Geometry check sheet. Reference: the model listing, model coordinates, mm. Face numbers are marked on the shaded views. Give positions to 0.01 mm unless a question says otherwise; leave off trailing zeros. Loops run counter-clockwise (first coordinate to the right, second up) from the corner with the lowest first, then second, coordinate; pieces in that order, holes last.
1. Release check for a two-part mould opening along Z. For the marked faces 1, 2 and 3 record: +Z half, -Z half, draft (parallel to the pull), parting line (faces both ways), or undercut.
2. Material ranges on L1, parallel to Z at x = -1.25, y = -1.7; L2, parallel to X at y = -4.65, z = -1.75; L3, parallel to Z at x = 0, y = -3.35, recorded low to high.
3. Cross-section at B-B, the plane x = 0. Record the cut outline in (y, z), plus the area to 3 significant figures.
4. Go/stop test with flat-tipped pins: pin 1 Ø2 at (y, z) = (-1, -8.5) entering from -X; pin 2 Ø3 at (y, z) = (-4.5, 7) entering from +X; pin 3 Ø3 at (y, z) = (-2.5, -2) entering from -X. Record where each tip stops, or that it passes through.
5. Cross-section at A-A, the plane z = 0. Record the cut outline in (x, y), plus the area to 3 significant figures.
6. Cross-section at C-C, the plane y = -1.35. Record the cut outline in (x, z), plus the area to 3 significant figures.
7. Cross-section at D-D, the plane y = -5.15. Record the cut outline in (x, z).
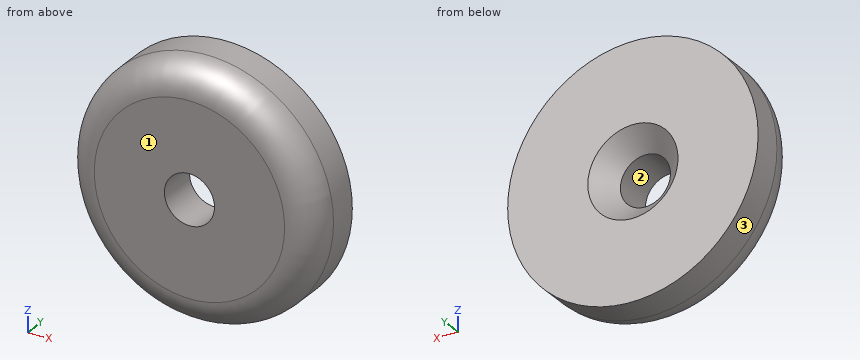
from build123d import *

# Parameters (mm, degrees)
F0_R     = 12.5
F0_R_2   = 2.5
F1_DEPTH = 6
F2_R     = 3
F3_SIZE  = 2


with BuildPart() as f1:
    # F0 (on Front) → F1 (new body)
    with BuildSketch(Plane.XZ):
        Circle(F0_R)
        Circle(F0_R_2, mode=Mode.SUBTRACT)
    extrude(amount=F1_DEPTH)

    # F2
    f2_edges = [f1.edges().sort_by_distance(p)[0] for p in [
        (-12.5, -6, 0),
    ]]
    fillet(f2_edges, radius=F2_R)

    # F3
    f3_edges = [f1.edges().sort_by_distance(p)[0] for p in [
        (-2.5, 0, 0),
    ]]
    chamfer(f3_edges, length=F3_SIZE)


solid = f1.part
Result:
1. face 1: draft
1. face 2: undercut
1. face 3: parting line
2. L1: z = -12.44 to -2.51, 2.51 to 12.44
2. L2: x = -11.88 to -1.79, 1.79 to 11.88
2. L3: z = -12.48 to -2.5, 2.5 to 12.48
3. outline: (-6, -9.5) arc R3 ccw to (-3, -12.5) - (0, -12.5) - (0, -4.5) - (-2, -2.5) - (-6, -2.5) - close; (-6, 2.5) - (-2, 2.5) - (0, 4.5) - (0, 12.5) - (-3, 12.5) arc R3 ccw to (-6, 9.5) - close
3. area: 112 mm2
4. pin 1: stops at x = -10
4. pin 2: stops at x = 11.02
4. pin 3: stops at x = -12.49
5. outline: (-12.5, -3) arc R3 ccw to (-9.5, -6) - (-2.5, -6) - (-2.5, -2) - (-4.5, 0) - (-12.5, 0) - close; (2.5, -6) - (9.5, -6) arc R3 ccw to (12.5, -3) - (12.5, 0) - (4.5, 0) - (2.5, -2) - close
5. area: 112 mm2
6. outline: circle Ø25 at (0, 0); hole circle Ø6.3 at (0, 0)
6. area: 460 mm2
7. outline: circle Ø23.18 at (0, 0); hole circle Ø5 at (0, 0)
